from build123d import *

# Parameters (mm, degrees)
SKETCH_1_R          = 16.5
SKETCH_1_R_2        = 2.05
EXTRUDE_1_DEPTH     = 7.6
SKETCH_2_R          = 3.225
CUT_EXTRUDE_1_DEPTH = 4


with BuildPart() as part:
    # 草图1 → 凸台-拉伸1 (new body)
    with BuildSketch(Plane(origin=(0, 0, 0), x_dir=(0, 0, -1), z_dir=(1, 0, 0))):
        with Locations(Location((0, 0, 0), (0, 0, 180))):
            Circle(SKETCH_1_R)
        with Locations(Location((0, 12, 0), (0, 0, 180))):
            Circle(SKETCH_1_R_2, mode=Mode.SUBTRACT)
        with Locations(Location((10.392304845, 6, 0), (0, 0, 180))):
            Circle(SKETCH_1_R_2, mode=Mode.SUBTRACT)
        with Locations(Location((10.392304845, -6, 0), (0, 0, 180))):
            Circle(SKETCH_1_R_2, mode=Mode.SUBTRACT)
        with Locations(Location((0, -12, 0), (0, 0, 180))):
            Circle(SKETCH_1_R_2, mode=Mode.SUBTRACT)
        with Locations(Location((-10.392304845, -6, 0), (0, 0, 180))):
            Circle(SKETCH_1_R_2, mode=Mode.SUBTRACT)
        with Locations(Location((-10.392304845, 6, 0), (0, 0, 180))):
            Circle(SKETCH_1_R_2, mode=Mode.SUBTRACT)
    extrude(amount=EXTRUDE_1_DEPTH)

    # 草图2 → 切除-拉伸1 (cut)
    with BuildSketch(Plane.ZY):
        Circle(SKETCH_2_R)
    extrude(amount=-CUT_EXTRUDE_1_DEPTH, mode=Mode.SUBTRACT)


solid = part.part
Check sheet for the modelled part. Datum: model origin and axes. Units: mm. A direction names the side the tool comes from. Give positions to 0.01 mm unless a question says otherwise; leave off trailing zeros. Write each loop counter-clockwise with the first axis right and the second up, starting at its lowest first coordinate (ties: lowest second). Pieces come first, ordered by that corner, then holes. Notation, with made-up numbers: (21, -16.75) -> (51, -16.75) arc R26 ccw to (51, 21.25) -> close; hole circle Ø5 at (86, 61). An arc over 180 degrees is marked (long way). Use one line per item in the form item = value. Start each with the question number.
1. Go/stop test with flat-tipped pins: P1, Ø3.5, axis at y = -12, z = 0, coming from the -X side; P2, Ø3, axis at x = 2, y = -8, coming from the -Z side; P3, Ø1, axis at x = 3.5, y = 2.5, coming from the +Z side; P4, Ø4, axis at x = 6, z = -9.5, coming from the -Y side. Record where each tip stops, or that it passes through.
2. Thickness scan on line 1 along Y through (x, z) = (1.5, 0) (3 decimals); line 2 along Z through (x, y) = (1.5, 7); line 3 along Y through (x, z) = (3.5, -11.5). Record the ranges inside material, lowest first. Write a range as from..to.
3. Mould release check, pull along Z, two halves, no side actions. Record for faces 1 (the cylindrical face through (3.747, -4.956, 15.738)), 2 (the flat face through (0, 3.4, -0.2)), 3 (the cylindrical face through (3.747, -9.999, -0.444)): pulls with the +Z half, pulls with the -Z half, needs draft (parallel to the pull), parting line crosses it, or undercut.
4. Section check B-B (y = 6). Record the cut outline in (x, z), and give its area (3 significant figures).
5. Section check D-D (x = 1.75). Record the cut outline in (y, z) (3 decimals).
6. Access from +Z, -Z, +X, -X, +Y, -Y to the whole of each face (thin tool, end or side, straight path). Record for faces 4 (the cylindrical face through (1.97, -3.15, -0.7)), 5 (the cylindrical face through (3.747, 7.247, -12.019)).
7. Section check C-C (z = -10.5). Record the cut outline in (x, y).
8. Section check A-A (x = 5.75). Record the cut outline in (y, z).
Conclusion:
q1.P1 = through
q1.P2 = -15.17
q1.P3 = 16.38
q1.P4 = -14.7
q2.line_1 = -16.5..-14.05, -9.95..-3.225, 3.225..9.95, 14.05..16.5
q2.line_2 = -14.94..-12.18, -8.6..8.6, 12.18..14.94
q2.line_3 = -11.83..-7.72, -4.28..4.28, 7.72..11.83
q3.face_1 = parting line crosses it
q3.face_2 = needs draft
q3.face_3 = undercut
q4.outline = (0, -15.37) -> (7.6, -15.37) -> (7.6, -12.44) -> (0, -12.44) -> close; (0, -8.34) -> (7.6, -8.34) -> (7.6, 8.34) -> (0, 8.34) -> close; (0, 12.44) -> (7.6, 12.44) -> (7.6, 15.37) -> (0, 15.37) -> close
q4.area = 171 mm²
q5.outline = circle Ø33 at (0, 0); hole circle Ø4.1 at (-12, 0); hole circle Ø4.1 at (-6, -10.392); hole circle Ø4.1 at (-6, 10.392); hole circle Ø6.45 at (0, 0); hole circle Ø4.1 at (6, -10.392); hole circle Ø4.1 at (6, 10.392); hole circle Ø4.1 at (12, 0)
q6.face_4 = -X
q6.face_5 = +X, -X
q7.outline = (0, -12.73) -> (7.6, -12.73) -> (7.6, -8.05) -> (0, -8.05) -> close; (0, -3.95) -> (7.6, -3.95) -> (7.6, 3.95) -> (0, 3.95) -> close; (0, 8.05) -> (7.6, 8.05) -> (7.6, 12.73) -> (0, 12.73) -> close
q8.outline = circle Ø33 at (0, 0); hole circle Ø4.1 at (-12, 0); hole circle Ø4.1 at (-6, -10.39); hole circle Ø4.1 at (-6, 10.39); hole circle Ø4.1 at (6, -10.39); hole circle Ø4.1 at (6, 10.39); hole circle Ø4.1 at (12, 0)
